```python
from build123d import *

# Parameters (mm, degrees)
F0_R     = 7.6601757708
F1_DEPTH = 20
F2_W     = 14.7302162368
F2_H     = 5.6654675864
F3_DEPTH = 25
F4_R     = 5.1556537043
F5_DEPTH = 38.2


# Not quite as in the source:
# - a feature of the source that left no trace in its solid (it failed there, or was rolled back) is left out


with BuildPart() as f1:
    # F0 (on Right) → F1 (new body)
    with BuildSketch(Plane.YZ):
        Circle(F0_R)
    extrude(amount=F1_DEPTH)

    # F2 (on Top) → F3 (join)
    with BuildSketch(Plane.XY):
        with Locations((9.9145689746, -0.1416367013)):
            Rectangle(F2_W, F2_H)
    extrude(amount=-F3_DEPTH)

    # F4 (on Right) → F5 (cut)
    with BuildSketch(Plane.YZ):
        Circle(F4_R)
    extrude(amount=F5_DEPTH, mode=Mode.SUBTRACT)


solid = f1.part
```
Part model, mm, in its own coordinate system. A direction names the side the tool comes from. Coordinates: 2 decimals unless noted, no trailing zeros. Order: outer loops, then holes, each group sorted by start corner. A loop starts at its lowest first (then second) coordinate and runs counter-clockwise, first axis right, second up. Notation, with made-up numbers: (5.25, -5) -> (38.25, -5) arc R22 cw to (38.25, 5) -> close; hole circle Ø1 at (14.5, 43.5). An arc over 180 degrees is marked (long way). Put each result on its own line as item: value. Start each with the question number.
(1) Mould opens along Z. For faces 4 (the face through (10, 0, -25)), 5 (the face through (0, 5, -2)), 6 (the face through (9.86, -0.67, 5.11)) say: pulls with the +Z half, pulls with the -Z half, needs draft (parallel to the pull), parting line crosses it, or undercut.
(2) Which spindle directions (+Z, -Z, +X, -X, +Y, -Y) get a long thin tool onto all of the face, cutting with end or side? Do faces 1 (the face through (10, -2.974, -16)), 2 (the face through (10, 2.691, -16)), 3 (the face through (20, 5, -2)). Say none if no direction does.
(3) Pin check, flat tips, straight feed: pin 1 Ø12 at (x, z) = (11.5, -20) entering from +Y; pin 2 Ø1 at (x, y) = (9, -5.5) entering from -Z; pin 3 Ø3 at (x, y) = (8.5, 5) entering from +Z; pin 4 Ø6 at (y, z) = (6, -11.5) entering from -X. Stop position of each tip, or through.
(4) Band-saw the part on D-D (z = -4.5). Give the cut face in (x, y).
(5) Band-saw the part on A-A (z = 0). Give the cut face in (x, y).
(6) Band-saw the part on B-B (y = 0). Give the cut face in (x, z), then the cut area to 3 significant figures.
(7) Probe line 1 along Z through (x, y) = (9.5, 0.25); line 2 along Z through (x, y) = (7, 0); line 3 along X through (y, z) = (1.5, -12). List the from-to ranges inside material, lowest first. Write a range as [from, to].
(8) Band-saw the part on C-C (x = 7.75). Give the cut face in (y, z), then the cut area to 3 significant figures.
Determined:
1. face 4: pulls with the -Z half
1. face 5: needs draft
1. face 6: undercut
2. face 1: -Z, +X, -X, -Y
2. face 2: -Z, +X, -X, +Y
2. face 3: +Z, -Z, +X, +Y, -Y
3. pin 1: stops at y = 2.69
3. pin 2: stops at z = -5.8
3. pin 3: stops at z = 6.81
3. pin 4: passes through
4. outline: (0, -6.2) -> (20, -6.2) -> (20, -2.52) -> (0, -2.52) -> close; (0, 2.52) -> (20, 2.52) -> (20, 6.2) -> (0, 6.2) -> close
5. outline: (0, -7.66) -> (20, -7.66) -> (20, -5.16) -> (0, -5.16) -> close; (0, 5.16) -> (20, 5.16) -> (20, 7.66) -> (0, 7.66) -> close
6. outline: (0, -7.66) -> (2.55, -7.66) -> (2.55, -25) -> (17.28, -25) -> (17.28, -7.66) -> (20, -7.66) -> (20, -5.16) -> (0, -5.16) -> close; (0, 5.16) -> (20, 5.16) -> (20, 7.66) -> (0, 7.66) -> close
6. area: 356 mm²
7. line 1: z = [-25, -5.15], [5.15, 7.66]
7. line 2: z = [-25, -5.16], [5.16, 7.66]
7. line 3: x = [2.55, 17.28]
8. outline: (-2.97, -25) -> (2.69, -25) -> (2.69, -7.17) arc R7.66 ccw (long way) to (-2.97, -7.06) -> close; hole circle Ø10.31 at (0, 0)
8. area: 200 mm²
